Model file for the job. Use its own axes, mm. Coordinates: 2 decimals unless noted, no trailing zeros. Write each loop counter-clockwise with the first axis right and the second up, starting at its lowest first coordinate (ties: lowest second). Pieces come first, ordered by that corner, then holes. Notation, with made-up numbers: M 14,4 L 65,4 A34 ccw 65,35 Z; hole C 57,8.25 d2. An arc over 180 degrees is marked long. Put each result on its own line as item: value. Start each with the question number.
Q1. Cut at C-C (x = 0.65). Write the cut outline in (y, z).
Q2. Cut at B-B (z = -122). Write the cut outline in (x, y).
Q3. Drill centre lines: line 1 along Y through (x, z) = (1.6, -109); line 2 along Z through (x, y) = (0.7, -180); line 3 along Y through (x, z) = (1.2, -203). Where is each one in solid material? Low to high.
Q4. Cut at D-D (z = -216). Write the cut outline in (x, y).
Q5. Cut at A-A (y = -216.5). Write the cut outline in (x, z).
```python
from build123d import *

# Parameters (mm, degrees)
SKETCH1_W           = 458
SKETCH1_H           = 476.6
BOSS_EXTRUDE1_DEPTH = 2
SKETCH2_W           = 51
SKETCH2_H           = 25
BOSS_EXTRUDE2_DEPTH = 2
SKETCH3_W           = 218.693705359
SKETCH3_H           = 52.165471003
CUT_EXTRUDE1_DEPTH  = 10


with BuildPart() as part:
    # Sketch1 → Boss-Extrude1 (new body)
    with BuildSketch(Plane(origin=(0, 0, 0), x_dir=(0, 0, -1), z_dir=(1, 0, 0))):
        with Locations((55.806722689, -22.770588235)):
            Rectangle(SKETCH1_W, SKETCH1_H)
    extrude(amount=BOSS_EXTRUDE1_DEPTH)

    # Sketch2 → Boss-Extrude2 (add)
    with BuildSketch(Plane(origin=(2, 0, 0), x_dir=(0, 0, -1), z_dir=(1, 0, 0))):
        with Locations((-147.693277311, -273.570588235)):
            Rectangle(SKETCH2_W, SKETCH2_H)
        with Locations((259.306722689, -273.570588235)):
            Rectangle(SKETCH2_W, SKETCH2_H)
    extrude(amount=-BOSS_EXTRUDE2_DEPTH)

    # Sketch3 → Cut-Extrude1 (cut)
    with BuildSketch(Plane.ZY):
        with Locations((-49.796656363, -205.571162235)):
            Rectangle(SKETCH3_W, SKETCH3_H)
    extrude(amount=-CUT_EXTRUDE1_DEPTH, mode=Mode.SUBTRACT)


solid = part.part
```
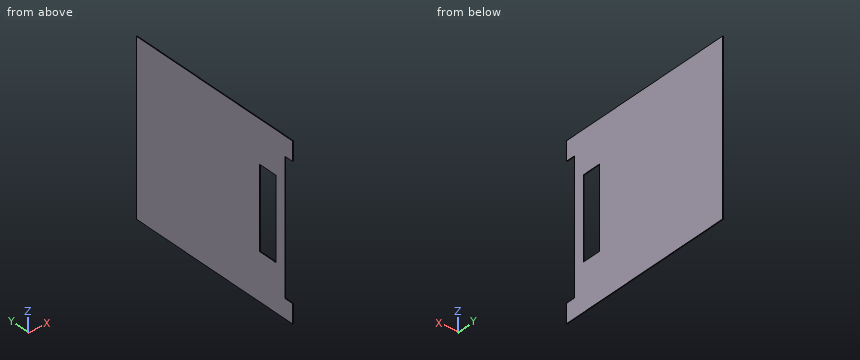
Computed values:
1. outline: M -286.07,-284.81 L 215.53,-284.81 L 215.53,173.19 L -286.07,173.19 L -286.07,122.19 L -261.07,122.19 L -261.07,-233.81 L -286.07,-233.81 Z; hole M -231.65,-159.14 L -179.49,-159.14 L -179.49,59.55 L -231.65,59.55 Z
2. outline: M 0,-261.07 L 2,-261.07 L 2,-231.65 L 0,-231.65 Z; M 0,-179.49 L 2,-179.49 L 2,215.53 L 0,215.53 Z
3. line 1: -261.07 to -231.65, -179.49 to 215.53
3. line 2: -284.81 to -159.14, 59.55 to 173.19
3. line 3: -261.07 to 215.53
4. outline: M 0,-261.07 L 2,-261.07 L 2,215.53 L 0,215.53 Z
5. outline: M 0,-284.81 L 2,-284.81 L 2,-159.14 L 0,-159.14 Z; M 0,59.55 L 2,59.55 L 2,173.19 L 0,173.19 Z
